```python
from build123d import *

# Parameters (mm, degrees)
SKETCH1_W           = 171.45
SKETCH1_H           = 20
BOSS_EXTRUDE1_DEPTH = 6
SKETCH2_W           = 19.55
SKETCH2_H           = 15
CUT_EXTRUDE1_DEPTH  = 3
SKETCH3_W           = 19.55
SKETCH3_H           = 5
CUT_EXTRUDE2_DEPTH  = 13
CHAMFER1_SIZE       = 1.8
SKETCH4_W           = 132.35
SKETCH4_H           = 4
BOSS_EXTRUDE2_DEPTH = 8
CUT_EXTRUDE3_DEPTH  = 3
CHAMFER2_SIZE       = 1.5
FILLET1_R           = 8
FILLET2_R           = 5


with BuildPart() as part:
    # Sketch1 → Boss-Extrude1 (new body)
    with BuildSketch(Plane.XY):
        Rectangle(SKETCH1_W, SKETCH1_H)
    extrude(amount=BOSS_EXTRUDE1_DEPTH)

    # Sketch2 → Cut-Extrude1 (cut)
    with BuildSketch(Plane.XY.offset(6)):
        with Locations((-75.95, -2.5)):
            Rectangle(SKETCH2_W, SKETCH2_H)
        with Locations((75.95, -2.5)):
            Rectangle(SKETCH2_W, SKETCH2_H)
    extrude(amount=-CUT_EXTRUDE1_DEPTH, mode=Mode.SUBTRACT)

    # Sketch3 → Cut-Extrude2 (cut)
    with BuildSketch(Plane.XY.offset(6)):
        with Locations((-75.95, 7.5)):
            Rectangle(SKETCH3_W, SKETCH3_H)
        with Locations((75.95, 7.5)):
            Rectangle(SKETCH3_W, SKETCH3_H)
    extrude(amount=-CUT_EXTRUDE2_DEPTH, mode=Mode.SUBTRACT)

    # Chamfer1
    chamfer1_edges = [part.edges().sort_by_distance(p)[0] for p in [
        (-66.175, -2.5, 3),
        (66.175, -2.5, 3),
    ]]
    chamfer(chamfer1_edges, length=CHAMFER1_SIZE)

    # Sketch4 → Boss-Extrude2 (add)
    with BuildSketch(Plane.XY.offset(6)):
        with Locations((0, -8)):
            Rectangle(SKETCH4_W, SKETCH4_H)
    extrude(amount=BOSS_EXTRUDE2_DEPTH)

    # Sketch5 → Cut-Extrude3 (cut)
    with BuildSketch(Plane.XY.offset(6)):
        with BuildLine():
            Line((-54.175, -6), (54.175, -6))
            ThreePointArc((54.175, -6), (56.296320344, -5.121320344), (57.175, -3))
            Line((57.175, -3), (57.175, 3))
            ThreePointArc((57.175, 3), (56.296320344, 5.121320344), (54.175, 6))
            Line((54.175, 6), (-54.175, 6))
            ThreePointArc((-54.175, 6), (-56.296320344, 5.121320344), (-57.175, 3))
            Line((-57.175, 3), (-57.175, -3))
            ThreePointArc((-57.175, -3), (-56.296320344, -5.121320344), (-54.175, -6))
        make_face()
    extrude(amount=-CUT_EXTRUDE3_DEPTH, mode=Mode.SUBTRACT)

    # Chamfer2
    chamfer2_edges = [part.edges().sort_by_distance(p)[0] for p in [
        (56.296320344, -5.121320344, 3),
        (0, -6, 3),
        (-56.296320344, -5.121320344, 3),
        (-57.175, 0, 3),
        (-56.296320344, 5.121320344, 3),
        (0, 6, 3),
        (56.296320344, 5.121320344, 3),
        (57.175, 0, 3),
    ]]
    chamfer(chamfer2_edges, length=CHAMFER2_SIZE)

    # Fillet1
    fillet1_edges = [part.edges().sort_by_distance(p)[0] for p in [
        (-85.725, -10, 1.5),
        (85.725, -10, 1.5),
    ]]
    fillet(fillet1_edges, radius=FILLET1_R)

    # Fillet2
    fillet2_edges = [part.edges().sort_by_distance(p)[0] for p in [
        (-66.175, -8, 14),
        (66.175, -8, 14),
    ]]
    fillet(fillet2_edges, radius=FILLET2_R)


solid = part.part
```
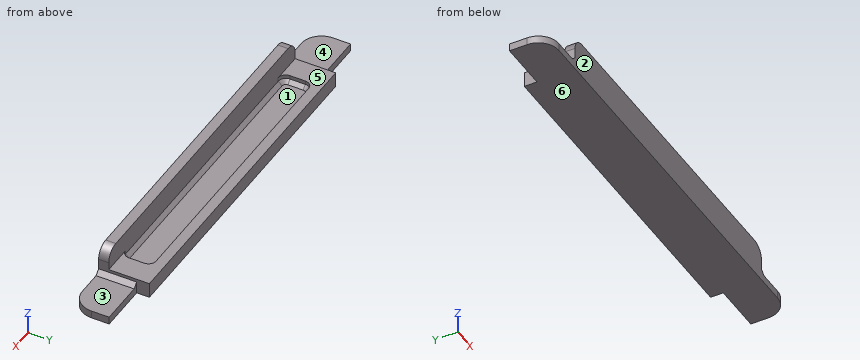
CAD build for the part. Positions are in the model's coordinates, mm. Face numbers are marked on the shaded views. A direction names the side the tool comes from. Round coordinates to 2 decimals unless told otherwise and drop trailing zeros. Order: outer loops, then holes, each group sorted by start corner. A loop starts at its lowest first (then second) coordinate and runs counter-clockwise, first axis right, second up. Notation, with made-up numbers: (29.5, 23.25) - (71.5, 23.25) arc R28 ccw to (71.5, 48.25) - close; hole circle Ø11 at (50, -13). An arc over 180 degrees is marked (long way). Answer in a Markdown table with one row per item. Add a question column.
(1) Band-saw the part on C-C on x = 1.5. List the corners of the cut face in (y, z).
(2) Band-saw the part on B-B on z = 1.5. List the corners of the cut face in (x, y) (3 decimals).
(3) Mould opens along Y. For the marked faces 1, 2 and 3 say: +Y half, -Y half, draft (parallel to the pull), parting line (faces both ways), or undercut.
(4) Band-saw the part on D-D on y = 7.5. List the corners of the cut face in (x, z) (3 decimals).
(5) 3-axis set-ups, long thin cutter, end or side, ignore diameter. For the marked faces 4, 5 and 6: which of +Z, -Z, +X, -X, +Y, -Y reach the whole face in a straight line?
(6) Band-saw the part on A-A on y = 0. List the corners of the cut face in (x, z) (3 decimals).
(7) Probe L1, parallel to Y at x = 11.5, z = 4.5; L2, parallel to X at y = 9, z = 1.75 (3 decimals); L3, parallel to Z at x = 21, y = 3.25. List the from-to ranges inside material, lowest first. Write a range as [from, to].
(8) Drop flat-ended pins along their axis: pin 1 Ø1.5 at (x, y) = (-13.5, -3) entering from +Z; pin 2 Ø0.8 at (y, z) = (0.5, 5.5) entering from +X (3 decimals); pin 3 Ø0.8 at (y, z) = (-0.5, 5.5) entering from -X (3 decimals). Give the stop position or say it passes through.
Data:
| question | item | result |
|---|---|---|
| 1 | outline | (-10, 0) - (10, 0) - (10, 6) - (6, 6) - (6, 4.5) - (4.5, 3) - (-4.5, 3) - (-6, 4.5) - (-6, 14) - (-10, 14) - close |
| 2 | outline | (-85.725, -2) arc R8 ccw to (-77.725, -10) - (77.725, -10) arc R8 ccw to (85.725, -2) - (85.725, 5) - (66.175, 5) - (66.175, 10) - (-66.175, 10) - (-66.175, 5) - (-85.725, 5) - close |
| 3 | face 1 | undercut |
| 3 | face 2 | -Y half |
| 3 | face 3 | draft |
| 4 | outline | (-66.175, 0) - (66.175, 0) - (66.175, 6) - (-66.175, 6) - close |
| 5 | face 4 | +Z, -X, +Y, -Y |
| 5 | face 5 | +Z, +X, -X, +Y |
| 5 | face 6 | -Z, +X, -X, +Y, -Y |
| 6 | outline | (-85.725, 0) - (85.725, 0) - (85.725, 3) - (67.975, 3) - (66.175, 4.8) - (66.175, 6) - (57.175, 6) - (57.175, 4.5) - (55.675, 3) - (-55.675, 3) - (-57.175, 4.5) - (-57.175, 6) - (-66.175, 6) - (-66.175, 4.8) - (-67.975, 3) - (-85.725, 3) - close |
| 7 | L1 | y = [-10, -6], [6, 10] |
| 7 | L2 | x = [-66.175, 66.175] |
| 7 | L3 | z = [0, 3] |
| 8 | pin 1 | stops at z = 3 |
| 8 | pin 2 | stops at x = 66.175 |
| 8 | pin 3 | stops at x = -66.175 |
